CAD build for the part. Positions are in the model's coordinates, mm. A direction names the side the tool comes from. Give positions to 0.01 mm unless a question says otherwise; leave off trailing zeros. Order: outer loops, then holes, each group sorted by start corner. A loop starts at its lowest first (then second) coordinate and runs counter-clockwise, first axis right, second up. Notation, with made-up numbers: M 38,-16.75 L 85,-16.75 A15 ccw 85,-7.75 Z; hole C 43.25,22 d11. An arc over 180 degrees is marked long. Put each result on its own line as item: value. Start each with the question number.
1) Drill centre lines: line 1 (Z direction, x = -3.25, y = 3.75); line 2 (X direction, y = -1.5, z = -4.5); line 3 (Z direction, x = -1, y = -0.25). Where is each one in solid material? Low to high. Write a range as [from, to].
2) Tool access for faces 1 (the face through (3, 3, 0)), 2 (the face through (0, 0, -19.05)): list every direction of +Z, -Z, +X, -X, +Y, -Y with a clear straight run to the whole face (end or side of a thin tool).
3) Cut at C-C (z = -5.5). Write the cut outline in (x, y), and give its area (3 significant figures).
4) Pin check, flat tips, straight feed: pin 1 (1.5 mm diameter, centred on x = -1, z = -4.5, fed in from -Y); pin 2 (6 mm diameter, centred on y = 4.5, z = -8, fed in from +X); pin 3 (5 mm diameter, centred on y = 3, z = -14, fed in from +X). Stop position of each tip, or through.
5) Cut at B-B (y = -4.5). Write the cut outline in (x, z), and give its area (3 significant figures).
6) Cut at D-D (y = 3.5). Write the cut outline in (x, z).
Solid Edge part; units mm, degrees
sketch "Sketch1" plane through (0, 0, 0) normal (0, 0, 1) x (1, 0, 0)
  circle A0 centre (0, 0) radius 6.4452
extrude "Protrusion1" add sketch "Sketch1" along normal blind 4.7625
sketch "Sketch2" plane through (0, 0, 0) normal (0, 0, -1) x (1, 0, 0)
  circle A0 centre (0, 0) radius 3.175
extrude "Protrusion2" add sketch "Sketch2" along normal blind 19.05
sketch "Sketch3" plane through (0, 0, -19.05) normal (0, 0, -1) x (1, 0, 0)
  circle A0 centre (0, 0) radius 3.1747
extrude "Cutout1" cut sketch "Sketch3" against normal blind 19.0309 flip side to cut
sketch "Sketch4" plane through (0, 0, 4.7625) normal (0, 0, 1) x (1, 0, 0)
  line L0 (-3.2664, 5.5562) -> (3.2664, 5.5562)
extrude "Cutout2" cut sketch "Sketch4" against normal up to next material side at (0, 5.6062, 4.7625)
sketch "Sketch5" plane through (0, 0, 0) normal (1, 0, 0) x (0, 1, 0)
  line L0 (-0.7937, -19.05) -> (-3.1747, -14.926)
revolve "RevolvedCutout1" cut sketch "Sketch5" angle 360 about axis through (0, 0, -14.7796) along (0, 0, 1) material side at (0, -2.0275, -17.013)
pattern_circular "Pattern1" count 6 over 360 about axis through (0, 0, 4.7625) along (0, 0, 1) of "Cutout2"
properties part number "24101329"
Solution:
1. line 1: [0, 4.76]
1. line 2: [-2.8, 2.8]
1. line 3: [-18.64, 4.76]
2. face 1: -Z
2. face 2: -Z, +X, -X, +Y, -Y
3. outline: C 0,0 d6.35
3. area: 31.7 mm²
4. pin 1: y = -3.16
4. pin 2: x = 2.8
4. pin 3: x = 3.14
5. outline: M -3.82,0 L 3.82,0 L 3.82,4.76 L -3.82,4.76 Z
5. area: 36.4 mm²
6. outline: M -4.4,0 L 4.4,0 L 4.4,4.76 L -4.4,4.76 Z
